```python
from build123d import *

# Parameters (mm, degrees)
F1_DEPTH = 25.4
F2_R     = 4.72896
F3_DEPTH = 6.35


with BuildPart() as f1:
    # F0 (on Top) → F1 (new body)
    with BuildSketch(Plane.XY):
        Polygon((19.05, 50.8), (-19.05, 50.8), (-19.05, -50.8), (19.05, -50.8), (19.05, -29.146114), align=None)
        with BuildLine():
            Line((19.05, -50.8), (-19.05, -50.8))
            add(Edge.make_bspline(
                [(-19.05, -50.8), (-17.541779, -58.375139), (0, -63.247859), (19.156481, -63.5)],
                knots=[0, 0, 0, 0, 40.261957, 40.261957, 40.261957, 40.261957], degree=3))
            Line((19.156481, -63.5), (19.156481, -50.8))
            Line((19.156481, -50.8), (19.05, -50.8))
        make_face()
        with BuildLine():
            add(Edge.make_bspline(
                [(19.05, -29.146114), (21.634858, -42.782448), (37.790419, -50.8), (47.486834, -50.8)],
                knots=[0, 0, 0, 0, 35.742752, 35.742752, 35.742752, 35.742752], degree=3))
            Line((19.05, -29.146114), (19.05, -50.8))
            Line((19.05, -50.8), (19.156481, -50.8))
            Line((19.156481, -50.8), (47.486834, -50.8))
        make_face()
        Polygon((19.156481, -50.8), (19.156481, -63.5), (69.950667, -63.5), (69.950667, -50.8), (47.486834, -50.8), align=None)
    extrude(amount=F1_DEPTH)

    # F2 (on Top) → F3 (cut, symmetric)
    with BuildSketch(Plane.XY):
        with Locations((-5.404981, 37.472747)):
            Circle(F2_R)
    extrude(amount=F3_DEPTH, both=True, mode=Mode.SUBTRACT)


solid = f1.part
```
The listing builds one solid part. Answer for the finished solid, in the listing's coordinates (mm). A direction names the side the tool comes from. Round coordinates to 2 decimals unless told otherwise and drop trailing zeros. Write each loop counter-clockwise with the first axis right and the second up, starting at its lowest first coordinate (ties: lowest second). Pieces come first, ordered by that corner, then holes. Notation, with made-up numbers: (52, -38) -> (100, -38) arc R13 ccw to (100, -30) -> close; hole circle Ø9 at (-8, 18). An arc over 180 degrees is marked (long way). Write item = value, one per line.
1) Section A-A on x = 56 is taken. Write down the section's boundary in (y, z).
Check values:
outline = (-63.5, 0) -> (-50.8, 0) -> (-50.8, 25.4) -> (-63.5, 25.4) -> close
2) For a pull along X with two mould halves and no side action, classify faces 4 (the flat face through (-5, 38, 6.35)), 5 (the flat face through (5, -6, 0)), 6 (the flat face through (69.951, -57, 13)) as released by +X, released by -X, zero draft, split by the parting line, or undercut.
Check values:
face_4 = undercut
face_5 = zero draft
face_6 = released by +X
3) Given pin 1 (10 mm diameter, centred on x = 47, z = 8, fed in from +Y); pin 2 (10 mm diameter, centred on y = 14, z = 10, fed in from +X); pin 3 (4.5 mm diameter, centred on x = -6, y = 37, fed in from -Z); pin 4 (4 mm diameter, centred on x = 17.5, z = 6, fed in from -Y), each flat-ended and moving along its own axis, determine where each tip first touches the part or whether it passes through.
Check values:
pin_1 = -50.1
pin_2 = 19.05
pin_3 = 6.35
pin_4 = -63.5
4) Which of the six approach directions +Z, -Z, +X, -X, +Y, -Y give full straight-line access (tool end or side, diameter ignored) to faces 1 (the flat face through (19.05, 10, 13)), 2 (the cylindrical face through (-6.43, 32.856, 3.219)), 3 (the flat face through (-19.05, 1, 13))?
Check values:
face_1 = +Z, -Z, +X, +Y
face_2 = -Z
face_3 = +Z, -Z, -X, +Y, -Y
5) Section B-B on y = -2 is taken. Write down the section's boundary in (x, z), plus the area to 3 significant figures.
Check values:
outline = (-19.05, 0) -> (19.05, 0) -> (19.05, 25.4) -> (-19.05, 25.4) -> close
area = 968 mm²
6) Straight lines are drawn through the part: line 1 along X through (y, z) = (28, 6.75); line 2 along Y through (x, z) = (18, 8); line 3 along Y through (x, z) = (48.5, 6.75). For each, find the intervals that lie inside material, in ascending order. Write a range as [from, to].
Check values:
line_1 = [-19.05, 19.05]
line_2 = [-63.48, 50.8]
line_3 = [-63.5, -50.8]
